For this review, take the finished solid that the model builds, in its own axes (mm). Face numbers are marked on the shaded views. A direction names the side the tool comes from. Coordinates: 2 decimals unless noted, no trailing zeros. Write each loop counter-clockwise with the first axis right and the second up, starting at its lowest first coordinate (ties: lowest second). Pieces come first, ordered by that corner, then holes. Notation, with made-up numbers: (-14, 9.5) -> (1, 9.5) arc R22 ccw to (1, 28.5) -> close; hole circle Ø1 at (50.5, 4). An arc over 180 degrees is marked (long way). Put each result on its own line as item: value. Start each with the question number.
Item 1: Consider section B-B on x = -3.5. Give the boundary of the cut face in (y, z).
Item 2: Consider section C-C on z = 18.5. Give the boundary of the cut face in (x, y).
Item 3: Insertion check: P1, Ø5, axis at y = -5.5, z = 16, coming from the +X side; P2, Ø5.5, axis at x = -16.5, z = -8.5, coming from the -Y side; P3, Ø3.5, axis at x = -2.5, z = 18.5, coming from the +Y side; P4, Ø6.5, axis at x = -15, y = -6, coming from the +Z side. Each pin has a flat end and moves straight along its axis. Give the tip position at first contact, or say it passes through.
Item 4: Consider section A-A on z = -16.5. Give the boundary of the cut face in (x, y), and give its area (3 significant figures).
Item 5: To check wall thickness, follow L1, parallel to X at y = -3, z = -6; L2, parallel to Z at x = -2.5, y = -0.5; L3, parallel to Z at x = -23, y = -7.75. State the ranges of each line that lie inside material, in increasing order.
Item 6: The part is to be moulded in two halves that separate along Z. For the marked faces 1, 2, 3 and 4, say which applies: +Z half, -Z half, draft (parallel to the pull), parting line (faces both ways), or undercut.
Item 7: For the marked faces 5, 6 and 7, list the 3-axis set-ups (+Z, -Z, +X, -X, +Y, -Y) from which the entire face can be reached by the end or side of a thin tool; tool diameter is ignored.
Item 8: Consider section D-D on y = -4. Give the boundary of the cut face in (x, z).
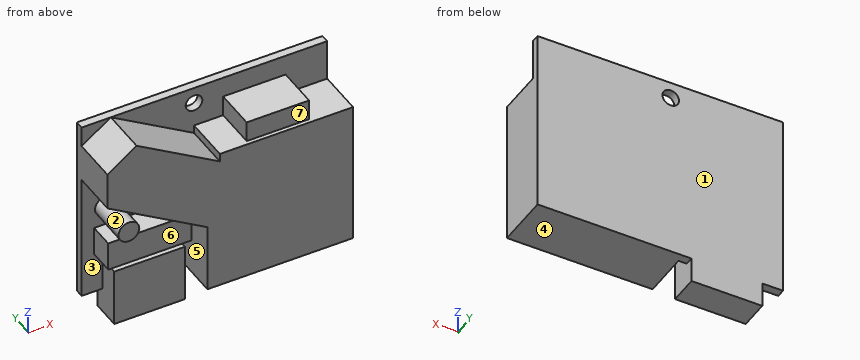
```python
from build123d import *

# Parameters (mm, degrees)
F0_W     = 17
F0_H     = 6
F1_DEPTH = 2
F3_DEPTH = 11
F2_W     = 15
F2_H     = 5
F4_DEPTH = 10
F5_D     = 4
F5_DEPTH = 6
F2_W_2   = 20
F2_H_2   = 7
F6_DEPTH = 6
F2_R     = 2.495167
F7_DEPTH = 10
F0_H_2   = 8
F8_DEPTH = 7


with BuildPart() as f1:
    # F0 (on Front) → F1 (new body)
    with BuildSketch(Plane.XZ):
        Polygon((29.5, 22.5), (-29.5, 22.5), (-29.5, -22.5), (-24.5, -22.5), (-24.5, -14.5), (-7.5, -14.5), (-7.5, -22.5), (29.5, -22.5), align=None)
        with Locations((-16, -25.5)):
            Rectangle(F0_W, F0_H)
    extrude(amount=F1_DEPTH)

    # F2 (on face) → F3 (join)
    with BuildSketch(Plane.XZ.offset(2)):
        Polygon((-2.5, 2.5), (-5.5, 2.5), (-5.5, -5.9), (-5.5, -22.5), (29.5, -22.5), (29.5, 2.5), align=None)
        Polygon((-5.5, -5.9), (-5.5, 2.5), (-2.5, 2.5), (-2.5, 10.5), (-5.5, 12.3), (-22.5, 22.5), (-29.5, 17.5), (-29.5, 8.5), align=None)
        Polygon((-2.5, 10.5), (-2.5, 2.5), (29.5, 2.5), (29.5, 12.5), (19.5, 12.5), (4.5, 12.5), (-2.5, 12.5), align=None)
    extrude(amount=F3_DEPTH)

    # F2 (on face) → F4 (join)
    with BuildSketch(Plane.XZ.offset(2)):
        with Locations((12, 15)):
            Rectangle(F2_W, F2_H)
    extrude(amount=F4_DEPTH)

    # F5
    with Locations(Plane.XZ.offset(2)):
        with Locations((-2.5, 18.5)):
            Hole(F5_D / 2, depth=F5_DEPTH)

    # F2 (on face) → F6 (join)
    with BuildSketch(Plane.XZ.offset(2)):
        with Locations((-16.5, -9)):
            Rectangle(F2_W_2, F2_H_2)
    extrude(amount=F6_DEPTH)

    # F2 (on face) → F7 (join)
    with BuildSketch(Plane.XZ.offset(2)):
        with Locations((-23.798013, -0.678133)):
            Circle(F2_R)
    extrude(amount=F7_DEPTH)

    # F0 (on Front) → F8 (join)
    with BuildSketch(Plane.XZ):
        with Locations((-16, -25.5)):
            Rectangle(F0_W, F0_H)
        with Locations((-16, -18.5)):
            Rectangle(F0_W, F0_H_2)
    extrude(amount=F8_DEPTH)


solid = f1.part
```
Return value:
1. outline: (-13, -22.5) -> (0, -22.5) -> (0, 16.77) -> (-2, 16.77) -> (-2, 11.1) -> (-13, 11.1) -> close; (-2, 20.23) -> (0, 20.23) -> (0, 22.5) -> (-2, 22.5) -> close
2. outline: (-29.5, -2) -> (-28.1, -2) -> (-28.1, -13) -> (-15.83, -13) -> (-15.83, -2) -> (-4.5, -2) -> (-4.5, 0) -> (-29.5, 0) -> close; (-0.5, -2) -> (29.5, -2) -> (29.5, 0) -> (-0.5, 0) -> close
3. P1: x = 19.5
3. P2: y = -8
3. P3: through
3. P4: z = 19.95
4. outline: (-29.5, -2) -> (-24.5, -2) -> (-24.5, -7) -> (-7.5, -7) -> (-7.5, -2) -> (-5.5, -2) -> (-5.5, -13) -> (29.5, -13) -> (29.5, 0) -> (-29.5, 0) -> close
4. area: 588 mm^2
5. L1: -26.5 to -6.5, -5.5 to 29.5
5. L2: -22.5 to 16.5, 20.5 to 22.5
5. L3: -12.5 to -5.5, -3.04 to 1.69, 4.6 to 22.14
6. face 1: draft
6. face 2: undercut
6. face 3: undercut
6. face 4: -Z half
7. face 5: -Z, -Y
7. face 6: -Z, -X, -Y
7. face 7: +Z, +X, -Y
8. outline: (-29.5, 8.5) -> (-5.5, -5.9) -> (-5.5, -22.5) -> (29.5, -22.5) -> (29.5, 12.5) -> (19.5, 12.5) -> (19.5, 17.5) -> (4.5, 17.5) -> (4.5, 12.5) -> (-2.5, 12.5) -> (-2.5, 10.5) -> (-22.5, 22.5) -> (-29.5, 17.5) -> close; (-26.5, -12.5) -> (-6.5, -12.5) -> (-6.5, -5.5) -> (-26.5, -5.5) -> close; circle Ø4.99 at (-23.8, -0.68); (-24.5, -28.5) -> (-7.5, -28.5) -> (-7.5, -14.5) -> (-24.5, -14.5) -> close
